Can you work these out from the model? Positions are in its coordinate system, mm. A direction names the side the tool comes from. Coordinates: 2 decimals unless noted, no trailing zeros. Loops run counter-clockwise (first coordinate to the right, second up) from the corner with the lowest first, then second, coordinate; pieces in that order, holes last.
```python
from build123d import *

# Parameters (mm, degrees)
F0_W     = 35.8
F0_H     = 59.3
F1_DEPTH = 32.3
F2_W     = 17.5
F2_H     = 19
F3_DEPTH = 1
F5_DEPTH = 2
F6_R     = 1.99999
F7_DEPTH = 1


# Not quite as in the source:
# - a fillet or chamfer is up to 0.001 mm smaller than in the source, because OpenCascade refuses the exact size


with BuildPart() as f1:
    # F0 (on Top) → F1 (new body)
    with BuildSketch(Plane.XY):
        Rectangle(F0_W, F0_H)
    extrude(amount=F1_DEPTH)

    # F2 (on face) → F3 (cut)
    with BuildSketch(Plane.XY.offset(32.3)):
        with Locations((0.45, -11.65)):
            Rectangle(F2_W, F2_H)
    extrude(amount=-F3_DEPTH, mode=Mode.SUBTRACT)

    # F4 (on face) → F5 (join)
    with BuildSketch(Plane(origin=(0, 29.65, 0), x_dir=(-1, 0, 0), z_dir=(0, 1, 0))):
        with BuildLine():
            ThreePointArc((4.3000000252, 32.3), (-1.9932503615, 17.1067496563), (13.2, 23.4))
            ThreePointArc((13.2, 23.4), (10.5932503615, 29.6932503437), (4.3000000252, 32.3))
        make_face()
    extrude(amount=F5_DEPTH)

    # F6 (radius 2 in the source; OpenCascade refuses exactly that, so slightly less here)
    f6_edges = [f1.edges().sort_by_distance(p)[0] for p in [
        (4.6, 31.65, 23.4),
    ]]
    fillet(f6_edges, radius=F6_R)

    # F7 (cut): a face of the model
    f7_faces = [f1.faces().sort_by_distance(p)[0] for p in [
        (-4.3, 31.65, 23.4),
    ]]
    extrude(f7_faces, amount=-F7_DEPTH, mode=Mode.SUBTRACT)


solid = f1.part
```
(1) I want a section at B-B on x = 13.5. Write out the boundary of the cut face in (y, z), then the cut area to 3 significant figures.
Check values:
outline: (-29.65, 0) - (29.65, 0) - (29.65, 32.3) - (-29.65, 32.3) - close
area: 1,920 mm2
(2) Which directions (+Z, -Z, +X, -X, +Y, -Y) give clear straight access to the entire face, cutting with the end or side of a thin tool? Please do faces 1 (the flat face through (-4, 30.65, 23)), 2 (the flat face through (0, 0, 0)).
Check values:
face 1: +Y
face 2: -Z, +X, -X, +Y, -Y
(3) I want a section at A-A on y = -7. Write out the boundary of the cut face in (x, z).
Check values:
outline: (-17.9, 0) - (17.9, 0) - (17.9, 32.3) - (9.2, 32.3) - (9.2, 31.3) - (-8.3, 31.3) - (-8.3, 32.3) - (-17.9, 32.3) - close
(4) I'm going to push flat-ended pins straight in: pin 1 (7 mm diameter, centred on x = -3, z = 26, fed in from +Y); pin 2 (1.1 mm diameter, centred on x = 0, z = 31.5, fed in from +Y). Where does each tip first touch, or does it pass through?
Check values:
pin 1: stops at y = 30.65
pin 2: stops at y = 30.67
(5) If we mould it in two halves opening along X, with no side actions, what happens to faces 3 (the flat face through (0, -12, 31.3)), 4 (the flat face through (0, -29.65, 16)), 5 (the flat face through (-17.9, 0, 16))? For each: released by +X, released by -X, zero draft, split by the parting line, or undercut.
Check values:
face 3: undercut
face 4: zero draft
face 5: released by -X
(6) I want a section at C-C on z = 13. Write out the boundary of the cut face in (x, y).
Check values:
outline: (-17.9, -29.65) - (17.9, -29.65) - (17.9, 29.65) - (-17.9, 29.65) - close
(7) If I drill on probe 1 along Z at (x, y) = (5, -18); probe 2 along Y at (x, z) = (3, 28); probe 3 along Y at (x, z) = (3.5, 3.5), over which ranges is the centre line in solid material (lowest first)?
Check values:
probe 1: z = 0 to 31.3
probe 2: y = -29.65 to 30.66
probe 3: y = -29.65 to 29.65
